Build history of the part. All positions in model axes, mm. A direction names the side the tool comes from. Give positions to 0.01 mm unless a question says otherwise; leave off trailing zeros. Order: outer loops, then holes, each group sorted by start corner. A loop starts at its lowest first (then second) coordinate and runs counter-clockwise, first axis right, second up. Notation, with made-up numbers: M 77,-9.5 L 118,-9.5 A17 cw 118,17.5 Z; hole C -36.5,-3.75 d3. An arc over 180 degrees is marked long. One line per item, written item: value.
from build123d import *

# Parameters (mm, degrees)
CROQUIS1_W              = 22.5
CROQUIS1_H              = 4
SALIENTE_EXTRUIR1_DEPTH = 3
CROQUIS5_W              = 4
CROQUIS5_H              = 31
CROQUIS5_R              = 1.05
SALIENTE_EXTRUIR3_DEPTH = 3
CROQUIS10_W             = 1.164205216
CROQUIS10_H             = 4.577506348
CORTAR_EXTRUIR4_DEPTH   = 42.716303767
CROQUIS3_R              = 1
SALIENTE_EXTRUIR4_DEPTH = 5
CROQUIS11_R             = 1.15
CORTAR_EXTRUIR5_DEPTH   = 42.907636536


with BuildPart() as part:
    # Croquis1 → Saliente-Extruir1 (new body)
    with BuildSketch(Plane.XY):
        with Locations((11.25, -2)):
            Rectangle(CROQUIS1_W, CROQUIS1_H)
    extrude(amount=SALIENTE_EXTRUIR1_DEPTH)

    # Croquis5 → Saliente-Extruir3 (add)
    with BuildSketch(Plane(origin=(0, 0, 0), x_dir=(-1, 0, 0), z_dir=(0, 0, -1))):
        with Locations((-2.75, -19.5)):
            Rectangle(CROQUIS5_W, CROQUIS5_H)
        with Locations((-2.75, -33)):
            Circle(CROQUIS5_R, mode=Mode.SUBTRACT)
    extrude(amount=-SALIENTE_EXTRUIR3_DEPTH)

    # Croquis10 → Cortar-Extruir4 (cut, through all)
    with BuildSketch(Plane.XY.offset(3)):
        with Locations((0.167897392, -1.711246826)):
            Rectangle(CROQUIS10_W, CROQUIS10_H)
    extrude(amount=-CORTAR_EXTRUIR4_DEPTH, mode=Mode.SUBTRACT)

    # Croquis3 → Saliente-Extruir4 (add)
    with BuildSketch(Plane(origin=(0, 0, 0), x_dir=(-1, 0, 0), z_dir=(0, 0, -1))):
        with Locations((-20, -2)):
            Circle(CROQUIS3_R)
    extrude(amount=-SALIENTE_EXTRUIR4_DEPTH)

    # Croquis11 → Cortar-Extruir5 (cut, through all)
    with BuildSketch(Plane(origin=(0, 0, 0), x_dir=(-1, 0, 0), z_dir=(0, 0, -1))):
        with Locations((-2.75, -33)):
            Circle(CROQUIS11_R)
    extrude(amount=-CORTAR_EXTRUIR5_DEPTH, mode=Mode.SUBTRACT)


solid = part.part
1) Saw through at A-A, the plane x = 2.75. Write the cut outline in (y, z), then the cut area to 3 significant figures.
Check values:
outline: M -35,0 L -34.15,0 L -34.15,3 L -35,3 Z; M -31.85,0 L 0,0 L 0,3 L -31.85,3 Z
area: 98.1 mm^2
2) Drill centre lines: probe 1 along Y at (x, z) = (2.75, 1.1); probe 2 along Y at (x, z) = (19, 2.45); probe 3 along X at (y, z) = (-32, 0.75). Where is each one in solid material? Low to high. Write a range as from..to.
Check values:
probe 1: -35..-34.15, -31.85..0
probe 2: -4..0
probe 3: 0.75..2.18, 3.32..4.75
3) Pin check, flat tips, straight feed: pin 1 (3 mm diameter, centred on x = 4.5, z = 1.5, fed in from +Y); pin 2 (1.5 mm diameter, centred on x = 12, z = 1.5, fed in from -Y); pin 3 (1.8 mm diameter, centred on x = 2.75, y = -33, fed in from +Z); pin 4 (1 mm diameter, centred on y = -15, z = 0.5, fed in from +X). Stop position of each tip, or through.
Check values:
pin 1: y = 0
pin 2: y = -4
pin 3: through
pin 4: x = 4.75
4) Saw through at B-B, the plane y = -33. Write the cut outline in (x, z).
Check values:
outline: M 0.75,0 L 1.6,0 L 1.6,3 L 0.75,3 Z; M 3.9,0 L 4.75,0 L 4.75,3 L 3.9,3 Z
5) Saw through at C-C, the plane z = 1.6. Write the cut outline in (x, y).
Check values:
outline: M 0.75,-35 L 4.75,-35 L 4.75,-4 L 22.5,-4 L 22.5,0 L 0.75,0 Z; hole C 2.75,-33 d2.3
6) Tool access for faces 1 (the face through (0.75, -18, 1)), 2 (the face through (4.75, -20, 1)): list every direction of +Z, -Z, +X, -X, +Y, -Y with a clear straight run to the whole face (end or side of a thin tool).
Check values:
face 1: +Z, -Z, -X, +Y, -Y
face 2: +Z, -Z, +X, -Y
7) Saw through at D-D, the plane y = -2. Write the cut outline in (x, z).
Check values:
outline: M 0.75,0 L 22.5,0 L 22.5,3 L 21,3 L 21,5 L 19,5 L 19,3 L 0.75,3 Z
8) Mould opens along X. For faces 3 (the face through (21, -2, 4)), 4 (the face through (2.999, -34.123, 1.479)), 5 (the face through (14, -4, 1)) say: released by +X, released by -X, zero draft, split by the parting line, or undercut.
Check values:
face 3: split by the parting line
face 4: undercut
face 5: zero draft
